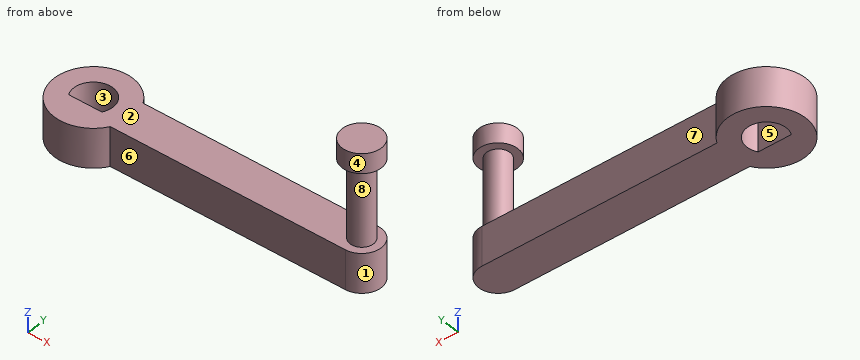
Autodesk Inventor part; units mm, degrees
ref_plane "YZ Plane" through (0, 0, 0) normal (1, 0, 0) x (0, 1, 0)
ref_plane "XZ Plane" through (0, 0, 0) normal (0, 1, 0) x (-1, 0, 0)
ref_plane "XY Plane" through (0, 0, 0) normal (0, 0, 1) x (1, 0, 0)
sketch "草圖2" plane through (0, 0, 0) normal (0, 0, 1) x (1, 0, 0)
  line L0 (4.3301, -2.5) -> (-4.3301, -2.5)
  arc A0 (4.3301, -2.5) -> (-4.3301, -2.5) centre (0, 0) ccw
  circle A1 centre (0, 0) radius 10
  line L1 (0, 0) -> (70, 0)
  circle A2 centre (70, 0) radius 5
  line L2 (8.6603, 5) -> (70, 5)
  line L3 (70, -5) -> (8.6603, -5)
  circle A3 centre (70, 0) radius 3
  dimension "d2" = 20
  dimension "d3" = 70
  dimension "d4" = 10
  dimension "d7" = 6
extrude "擠出1" add sketch "草圖2" against normal blind 10 contours A1 | A1 L2 A2 L1 | L1 A2 L3 A1 | A3 | A2
extrude "擠出2" add sketch "草圖2" along normal blind 20 contours A3
sketch "草圖3" plane through (70, 0, 20) normal (0, 0, 1) x (1, 0, 0)
  circle A0 centre (0, 0) radius 5
  point P0 (-70, 0)
  dimension "d10" = 10
extrude "擠出3" add sketch "草圖3" along normal blind 5
properties part number "Cranker1"
Design review of the part built by this model. Coordinates are the model's own, in mm. Face numbers are marked on the shaded views. A direction names the side the tool comes from. Give positions to 0.01 mm unless a question says otherwise; leave off trailing zeros. Loops run counter-clockwise (first coordinate to the right, second up) from the corner with the lowest first, then second, coordinate; pieces in that order, holes last. Notation, with made-up numbers: M 27,-2.5 L 73,-2.5 A11 ccw 73,10.5 Z; hole C 24,8 d1. An arc over 180 degrees is marked long. Write item = value, one per line.
Q1. For the marked faces 4, 5, 6, 7 and 8, list the 3-axis set-ups (+Z, -Z, +X, -X, +Y, -Y) from which the entire face can be reached by the end or side of a thin tool; tool diameter is ignored.
Output values:
face_4 = +Z
face_5 = +Z, -Z
face_6 = +Z, -Z, +X, -Y
face_7 = +Z, -Z, +X, +Y
face_8 = none
Q2. Draft analysis for pull direction X (two halves, no side actions). For the marked faces 1, 2 and 3, state which applies: +X half, -X half, draft (parallel to the pull), parting line (faces both ways), or undercut.
Output values:
face_1 = +X half
face_2 = draft
face_3 = undercut
Q3. We need section B-B (y = 0). Give the boundary of the cut face in (x, z).
Output values:
outline = M -10,-10 L -5,-10 L -5,0 L -10,0 Z; M 5,-10 L 75,-10 L 75,0 L 73,0 L 73,20 L 75,20 L 75,25 L 65,25 L 65,20 L 67,20 L 67,0 L 5,0 Z
Q4. To check wall thickness, follow line 1 (X direction, y = 0, z = -4); line 2 (Y direction, x = 0, z = -6.5); line 3 (Z direction, x = 67.5, y = -2.5). State the ranges of each line that lie inside material, in increasing order. Write a range as [from, to].
Output values:
line_1 = [-10, -5], [5, 75]
line_2 = [-10, -2.5], [5, 10]
line_3 = [-10, 0], [20, 25]
Q5. Insertion check: pin 1 (6 mm diameter, centred on x = 15, y = 4.5, fed in from +Z); pin 2 (6 mm diameter, centred on y = -0.5, z = -6, fed in from -X); pin 3 (8 mm diameter, centred on x = 43, z = -2.5, fed in from +Y); pin 4 (8 mm diameter, centred on x = 45, z = -5, fed in from -Y). Each pin has a flat end and moves straight along its axis. Give the tip position at first contact, or say it passes through.
Output values:
pin_1 = 0
pin_2 = -10
pin_3 = 5
pin_4 = -5
Q6. We need section D-D (x = 34.5). Give the boundary of the cut face in (y, z).
Output values:
outline = M -5,-10 L 5,-10 L 5,0 L -5,0 Z
Q7. We need section A-A (x = 0). Give the boundary of the cut face in (y, z), plus the area to 3 significant figures.
Output values:
outline = M -10,-10 L -2.5,-10 L -2.5,0 L -10,0 Z; M 5,-10 L 10,-10 L 10,0 L 5,0 Z
area = 125 mm^2
Q8. We need section C-C (z = 9). Give the boundary of the cut face in (x, y).
Output values:
outline = C 70,0 d6
